```python
from build123d import *

# Parameters (mm, degrees)
EXTRUDE_1_DEPTH = 35
SKETCH_2_R      = 1.25
EXTRUDE_2_DEPTH = 6


# Read off the part's stored shape, not the designer's step: M3 螺纹孔1
with BuildPart() as part:
    # 草图1 → 凸台-拉伸1 (new body)
    with BuildSketch(Plane.XY):
        Polygon((2.598076211, 0), (1.299038106, 2.25), (-1.299038106, 2.25), (-2.598076211, 0), (-1.299038106, -2.25), (1.299038106, -2.25), align=None)
    extrude(amount=EXTRUDE_1_DEPTH)

    # 草图2 → 凸台-拉伸2 (add)
    with BuildSketch(Plane.XY.offset(35)):
        Circle(SKETCH_2_R)
    extrude(amount=EXTRUDE_2_DEPTH)

    # M3 螺纹孔1 outline → M3 螺纹孔1 (revolve, cut)
    with BuildSketch(Plane.XZ):
        Polygon((1.25, 7.5), (0, 8.251075774), (0, 0), (1.25, 0), align=None)
    revolve(axis=Axis((0, 0, 0), (0, 0, 1)), mode=Mode.SUBTRACT)


solid = part.part
```
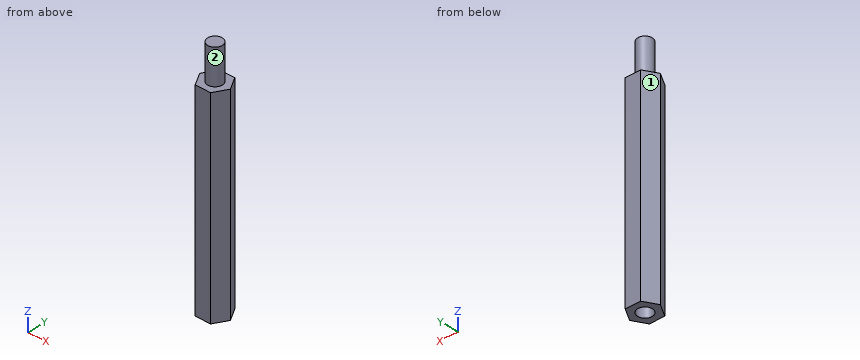
The model under review builds one solid part; all positions refer to its coordinate system, in mm. Face numbers are marked on the shaded views. A direction names the side the tool comes from. Give positions to 0.01 mm unless a question says otherwise; leave off trailing zeros. Write each loop counter-clockwise with the first axis right and the second up, starting at its lowest first coordinate (ties: lowest second). Pieces come first, ordered by that corner, then holes.
(1) To check wall thickness, follow L1, parallel to Z at x = 0.1, y = -2; L2, parallel to Y at x = 0, z = 2.5; L3, parallel to Y at x = 1.8, z = 12. State the ranges of each line that lie inside material, in increasing order.
(2) Consider section B-B, the plane y = 1.85. Give the boundary of the cut face in (x, z), and give its area (3 significant figures).
(3) Consider section A-A, the plane z = 19.5. Give the boundary of the cut face in (x, y).
(4) Tool access review of the marked faces 1 and 2: name each direction out of +Z, -Z, +X, -X, +Y, -Y from which nothing blocks a thin tool from reaching the whole face with its end or side.
Returned:
1. L1: z = 0 to 35
1. L2: y = -2.25 to -1.25, 1.25 to 2.25
1. L3: y = -1.38 to 1.38
2. outline: (-1.53, 0) - (1.53, 0) - (1.53, 35) - (-1.53, 35) - close
2. area: 107 mm2
3. outline: (-2.6, 0) - (-1.3, -2.25) - (1.3, -2.25) - (2.6, 0) - (1.3, 2.25) - (-1.3, 2.25) - close
4. face 1: +Z, -Z, -X, +Y
4. face 2: +Z
